For this review, take the finished solid that the model builds, in its own axes (mm). A direction names the side the tool comes from. Round coordinates to 2 decimals unless told otherwise and drop trailing zeros. Order: outer loops, then holes, each group sorted by start corner. A loop starts at its lowest first (then second) coordinate and runs counter-clockwise, first axis right, second up.
from build123d import *

# Parameters (mm, degrees)
SKETCH2_R           = 5
BOSS_EXTRUDE1_DEPTH = 4
FILLET1_R           = 1
CUT_EXTRUDE2_DEPTH  = 2.5
SKETCH4_R           = 3.125
BOSS_EXTRUDE3_DEPTH = 33
SKETCH5_R           = 3.125
SKETCH5_R_2         = 2
CUT_EXTRUDE4_DEPTH  = 6


with BuildPart() as part:
    # Sketch2 → Boss-Extrude1 (new body)
    with BuildSketch(Plane(origin=(0, 0, 0), x_dir=(0, 0, -1), z_dir=(1, 0, 0))):
        Circle(SKETCH2_R)
    extrude(amount=BOSS_EXTRUDE1_DEPTH)

    # Fillet1
    fillet1_edges = [part.edges().sort_by_distance(p)[0] for p in [
        (0, 0, 5),
    ]]
    fillet(fillet1_edges, radius=FILLET1_R)

    # Sketch3 → Cut-Extrude2 (cut)
    with BuildSketch(Plane.ZY):
        Polygon((2.075995504, 1.011719328), (0.161823113, 2.303724509), (-1.914172392, 1.292005181), (-2.075995504, -1.011719328), (-0.161823113, -2.303724509), (1.914172392, -1.292005181), align=None)
    extrude(amount=-CUT_EXTRUDE2_DEPTH, mode=Mode.SUBTRACT)

    # Sketch4 → Boss-Extrude3 (add)
    with BuildSketch(Plane(origin=(4, 0, 0), x_dir=(0, 0, -1), z_dir=(1, 0, 0))):
        Circle(SKETCH4_R)
    extrude(amount=BOSS_EXTRUDE3_DEPTH)

    # Sketch5 → Cut-Extrude4 (cut)
    with BuildSketch(Plane(origin=(37, 0, 0), x_dir=(0, 0, -1), z_dir=(1, 0, 0))):
        Circle(SKETCH5_R)
        Circle(SKETCH5_R_2, mode=Mode.SUBTRACT)
    extrude(amount=-CUT_EXTRUDE4_DEPTH, mode=Mode.SUBTRACT)


solid = part.part
(1) Tool access review of faces 1 (the face through (4, -3.3, 0.1)), 2 (the face through (2.48, -4.88, 1.08)), 3 (the face through (1.232, 1.805, -0.862)): name each direction out of +Z, -Z, +X, -X, +Y, -Y from which nothing blocks a thin tool from reaching the whole face with its end or side.
(2) Wall thickness on L1, parallel to X at y = 3.75, z = -0.5; L2, parallel to X at y = -1.5, z = -2.5; L3, parallel to Y at x = 8, z = -0.25: over which ranges is each line inside the solid? List them lowest first.
(3) Add section A-A on x = 19. Give the boundary of the cut face in (y, z) (3 decimals), plus the area to 3 significant figures.
(4) Clearance check with flat-ended pins moving along their axes: P1, Ø2, axis at x = 27.5, z = -2, coming from the +Y side; P2, Ø1, axis at y = 3.5, z = -3.5, coming from the +X side; P3, Ø4.5, axis at y = 0.5, z = -1, coming from the -X side; P4, Ø2, axis at x = 25.5, z = 3, coming from the +Y side. State where each tip first meets the part, or that it passes through.
(5) Draft analysis for pull direction Z (two halves, no side actions). For faces 4 (the face through (0, 2, -1)), 5 (the face through (1.23, -1.65, -1.13)), 6 (the face through (2.5, 0, 0)), 7 (the face through (17.31, 0.94, -2.98)), state which applies: pulls with the +Z half, pulls with the -Z half, needs draft (parallel to the pull), parting line crosses it, or undercut.
(6) Add section B-B on y = 0. Give the boundary of the cut face in (x, z) (3 decimals).
Here are the results:
1. face 1: +X
1. face 2: +X, -X
1. face 3: -X
2. L1: x = 0 to 4
2. L2: x = 0 to 31
2. L3: y = -3.11 to 3.11
3. outline: circle Ø6.25 at (0, 0)
3. area: 30.7 mm2
4. P1: stops at y = 2.96
4. P2: stops at x = 4
4. P3: stops at x = 0
4. P4: stops at y = 2.4
5. face 4: needs draft
5. face 5: undercut
5. face 6: undercut
5. face 7: parting line crosses it
6. outline: (0, -4) arc R1 ccw to (1, -5) - (4, -5) - (4, -3.125) - (31, -3.125) - (31, -2) - (37, -2) - (37, 2) - (31, 2) - (31, 3.125) - (4, 3.125) - (4, 5) - (1, 5) arc R1 ccw to (0, 4) - (0, 2.005) - (2.5, 2.005) - (2.5, -2.005) - (0, -2.005) - close
